Geometry check sheet. Reference: the model listing, model coordinates, mm. A direction names the side the tool comes from. Coordinates: 2 decimals unless noted, no trailing zeros. Order: outer loops, then holes, each group sorted by start corner. A loop starts at its lowest first (then second) coordinate and runs counter-clockwise, first axis right, second up. Notation, with made-up numbers: (53, 24) - (79, 24) arc R4 cw to (79, 28) - close; hole circle Ø4 at (30, 55.25). An arc over 180 degrees is marked (long way). Return JSON: item names as keys, results as strings. Group by question number.
Item 1: Section check C-C on y = 56. Enter the section's corners in (x, z).
Item 2: Section check A-A on x = 0. Enter the section's corners in (y, z).
Item 3: Section check B-B on z = 0. Enter the section's corners in (x, y).
Item 4: Section check D-D on x = 6. Enter the section's corners in (y, z), then the cut area to 3 significant figures.
Item 5: Scan lines: probe 1 along Y at (x, z) = (1, 6); probe 2 along Y at (x, z) = (-15, -2); probe 3 along Z at (x, y) = (-11, 62.5). Record each from-to range of solid material in increasing order.
Item 6: Gauge pin test, flat ends, axial feed: pin 1 (10 mm diameter, centred on x = -2.5, z = -12.5, fed in from +Y); pin 2 (2.5 mm diameter, centred on y = 89, z = 0, fed in from -X); pin 3 (3.5 mm diameter, centred on x = 9.5, z = -10, fed in from +Y). Record the tip position at first contact, or that the pin passes through.
Item 7: Tool access check on faces 1 (the flat face through (0, 0, 0)), 2 (the flat face through (-3, 92, 0)), 3 (the cylindrical face through (10.706, 77.642, 8.635)). Record the directions out of +Z, -Z, +X, -X, +Y, -Y that give a thin tool (end or side, any length) a straight path to the whole face; none if there is none.
Item 8: Draft check along Z on faces 4 (the flat face through (10, 74.6, 10)), 5 (the flat face through (0, 82.6, 5)), 6 (the flat face through (-19, 26, 20)), 7 (the cylindrical face through (9.574, 77.642, -8.435)). Enter one of: pulls with the +Z half, pulls with the -Z half, needs draft (parallel to the pull), parting line crosses it, or undercut.
Autodesk Inventor part; units mm, degrees
ref_plane "YZ Plane" through (0, 0, 0) normal (1, 0, 0) x (0, 1, 0)
ref_plane "XZ Plane" through (0, 0, 0) normal (0, 1, 0) x (-1, 0, 0)
ref_plane "XY Plane" through (0, 0, 0) normal (0, 0, 1) x (1, 0, 0)
sketch "草圖1" plane through (0, 0, 0) normal (0, 1, 0) x (-1, 0, 0)
  line L0 (18, 21) -> (-18, 21)
  line L1 (-21, 18) -> (-21, -18)
  line L2 (-18, -21) -> (18, -21)
  line L3 (21, -18) -> (21, 18)
  line L4 (21, 21) -> (-21, -21) construction
  line L5 (-21, 21) -> (21, -21) construction
  line L6 (21, -18) -> (18, -21)
  line L7 (-18, -21) -> (-21, -18)
  line L8 (-21, 18) -> (-18, 21)
  line L9 (18, 21) -> (21, 18)
  point P0 (0, 0)
  dimension "d0" = 42
  dimension "d1" = 42
  dimension "d2" = 3
  dimension "d3" = 3
  dimension "d4" = 3
  dimension "d5" = 3
  dimension "d6" = 3
  dimension "d7" = 3
  dimension "d8" = 3
  dimension "d9" = 3
extrude "擠出1" add sketch "草圖1" along normal blind 52.6
sketch "草圖2" plane through (0, 52.6, 0) normal (0, 1, 0) x (1, 0, 0)
  circle A0 centre (0, 0) radius 18
  dimension "d12" = 36
extrude "擠出2" add sketch "草圖2" along normal blind 28
sketch "草圖3" plane through (0, 80.6, 0) normal (0, 1, 0) x (1, 0, 0)
  circle A0 centre (0, 0) radius 14 construction
  circle A1 centre (0, 0) radius 11
  line L0 (0, 0) -> (-19.5, -19.5) construction
  line L1 (-21, -18) -> (-18, -21)
  circle A2 centre (-9.8995, -9.8995) radius 1.5
  circle A3 centre (9.8995, -9.8995) radius 1.5
  circle A4 centre (9.8995, 9.8995) radius 1.5
  circle A5 centre (-9.8995, 9.8995) radius 1.5
  dimension "d15" = 28
  dimension "d16" = 22
  dimension "d18" = 3
  dimension "d21" = 360
extrude "擠出3" cut sketch "草圖3" against normal blind 6 contours A2 | A3 | A4 | A5
extrude "擠出4" add sketch "草圖3" along normal blind 2 contours A1
sketch "草圖4" plane through (0, 82.6, 0) normal (0, 1, 0) x (1, 0, 0)
  circle A0 centre (0, 0) radius 4
  dimension "d27" = 8
extrude "擠出5" add sketch "草圖4" along normal blind 17
sketch "草圖5" plane through (0, 99.6, 0) normal (0, 1, 0) x (1, 0, 0)
  circle A0 centre (0, 0) radius 4
  line L0 (-3, -2.6458) -> (-3, 2.6458)
  dimension "d30" = 7
extrude "擠出6" cut sketch "草圖5" against normal blind 15 contours L0 A0 picked at (-3.1815, -0.6179)
sketch "草圖7" plane through (0, 0, 0) normal (0, -1, 0) x (1, 0, 0)
  point P0 (0, 0)
  point P1 (0, 0)
equation "\"d3\" = d2"
equation "\"d4\" = d2"
equation "\"d5\" = d4"
equation "\"d6\" = d2"
equation "\"d7\" = d6"
equation "\"d8\" = d2"
equation "\"d9\" = d8"
properties part number "stepper 42-27"
Computed:
{
 "1": {"outline": "circle Ø36 at (0, 0)"},
 "2": {"outline": "(0, -21) - (52.6, -21) - (52.6, -18) - (80.6, -18) - (80.6, -11) - (82.6, -11) - (82.6, -4) - (99.6, -4) - (99.6, 4) - (82.6, 4) - (82.6, 11) - (80.6, 11) - (80.6, 18) - (52.6, 18) - (52.6, 21) - (0, 21) - close"},
 "3": {"outline": "(-21, 0) - (21, 0) - (21, 52.6) - (18, 52.6) - (18, 80.6) - (11, 80.6) - (11, 82.6) - (4, 82.6) - (4, 99.6) - (-3, 99.6) - (-3, 84.6) - (-4, 84.6) - (-4, 82.6) - (-11, 82.6) - (-11, 80.6) - (-18, 80.6) - (-18, 52.6) - (-21, 52.6) - close"},
 "4": {"outline": "(0, -21) - (52.6, -21) - (52.6, -16.97) - (80.6, -16.97) - (80.6, -9.22) - (82.6, -9.22) - (82.6, 9.22) - (80.6, 9.22) - (80.6, 16.97) - (52.6, 16.97) - (52.6, 21) - (0, 21) - close", "area": "3,200 mm²"},
 "5": {"probe 1": "y = 0 to 82.6", "probe 2": "y = 0 to 80.6", "probe 3": "z = -14.25 to 14.25"},
 "6": {"pin 1": "stops at y = 82.6", "pin 2": "stops at x = -3", "pin 3": "stops at y = 80.6"},
 "7": {"face 1": "+Z, -Z, +X, -X, -Y", "face 2": "+Z, -Z, -X, +Y", "face 3": "+Y"},
 "8": {"face 4": "undercut", "face 5": "needs draft", "face 6": "pulls with the +Z half", "face 7": "undercut"}
}
